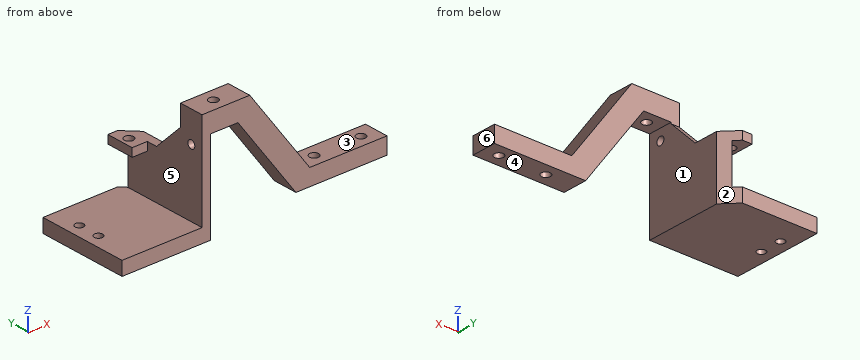
```python
from build123d import *

# Parameters (mm, degrees)
SZKIC1_W                    = 28
SZKIC1_H                    = 9
SZKIC1_R                    = 1.65
DODANIE_WYCI_GNI_CIE1_DEPTH = 6
DODANIE_WYCI_GNI_CIE2_DEPTH = 9
SZKIC3_W                    = 3
SZKIC3_H                    = 40.009031977
DODANIE_WYCI_GNI_CIE3_DEPTH = 9
SZKIC10_R                   = 1.65
WYTNIJ_WYCI_GNI_CIE4_DEPTH  = 7
SZKIC11_W                   = 32
SZKIC11_H                   = 33
SZKIC11_R                   = 1.5
DODANIE_WYCI_GNI_CIE4_DEPTH = 5
SZKIC12_W                   = 3
SZKIC12_H                   = 17.504515989
DODANIE_WYCI_GNI_CIE5_DEPTH = 24
SZKIC13_W                   = 10
SZKIC13_H                   = 3
DODANIE_WYCI_GNI_CIE6_DEPTH = 33
SZKIC14_R                   = 1.65
WYTNIJ_WYCI_GNI_CIE5_DEPTH  = 3
SZKIC15_W                   = 7
SZKIC15_H                   = 22.85
WYTNIJ_WYCI_GNI_CIE6_DEPTH  = 3
SFAZOWANIE1_SIZE            = 10
SZKIC16_R                   = 1.5
WYTNIJ_WYCI_GNI_CIE7_DEPTH  = 5
SZKIC17_R                   = 1.46285789
WYTNIJ_WYCI_GNI_CIE8_DEPTH  = 3
SZKIC18_W                   = 3
SZKIC18_H                   = 10.15
WYTNIJ_WYCI_GNI_CIE9_DEPTH  = 1.5
WYTNIJ_WYCI_GNI_CIE10_REACH = 87.52


with BuildPart() as part:
    # Szkic1 → Dodanie-wyciągnięcie1 (new body)
    with BuildSketch(Plane.XY):
        with Locations((14, 4.5)):
            Rectangle(SZKIC1_W, SZKIC1_H)
        with Locations((5.5, 4.5)):
            Circle(SZKIC1_R, mode=Mode.SUBTRACT)
        with Locations((22.5, 4.5)):
            Circle(SZKIC1_R, mode=Mode.SUBTRACT)
    extrude(amount=DODANIE_WYCI_GNI_CIE1_DEPTH)

    # Szkic2 → Dodanie-wyciągnięcie2 (add)
    with BuildSketch(Plane.XZ):
        Polygon((0, 0), (-5, 0), (-26, 29.009031977), (-36, 29.009031977), (-36, 36.009031977), (-21.72391247, 36.009031977), (0, 6), align=None)
    extrude(amount=-DODANIE_WYCI_GNI_CIE2_DEPTH)

    # Szkic3 → Dodanie-wyciągnięcie3 (add)
    with BuildSketch(Plane.XZ):
        with Locations((-37.5, 16.004515988)):
            Rectangle(SZKIC3_W, SZKIC3_H)
    extrude(amount=-DODANIE_WYCI_GNI_CIE3_DEPTH)

    # Szkic10 → Wytnij-wyciągnięcie4 (cut)
    with BuildSketch(Plane.XY.offset(36.009031977)):
        with Locations((-31, 4.5)):
            Circle(SZKIC10_R)
    extrude(amount=-WYTNIJ_WYCI_GNI_CIE4_DEPTH, mode=Mode.SUBTRACT)

    # Szkic11 → Dodanie-wyciągnięcie4 (add)
    with BuildSketch(Plane(origin=(0, 0, -4), x_dir=(-1, 0, 0), z_dir=(0, 0, -1))):
        with Locations((52, 16.5)):
            Rectangle(SZKIC11_W, SZKIC11_H)
        with Locations((63.5, 15)):
            Circle(SZKIC11_R, mode=Mode.SUBTRACT)
    extrude(amount=-DODANIE_WYCI_GNI_CIE4_DEPTH)

    # Szkic12 → Dodanie-wyciągnięcie5 (add)
    with BuildSketch(Plane(origin=(0, 9, 0), x_dir=(1, 0, 0), z_dir=(0, 1, 0))):
        with Locations((-37.5, -9.752257995)):
            Rectangle(SZKIC12_W, SZKIC12_H)
    extrude(amount=DODANIE_WYCI_GNI_CIE5_DEPTH)

    # Szkic13 → Dodanie-wyciągnięcie6 (add)
    with BuildSketch(Plane(origin=(0, 33, 0), x_dir=(1, 0, 0), z_dir=(0, 1, 0))):
        with Locations((-41, -17.004515989)):
            Rectangle(SZKIC13_W, SZKIC13_H)
    extrude(amount=-DODANIE_WYCI_GNI_CIE6_DEPTH)

    # Szkic14 → Wytnij-wyciągnięcie5 (cut)
    with BuildSketch(Plane.XY.offset(18.504515989)):
        with Locations((-41.65, 27.5)):
            Circle(SZKIC14_R)
    extrude(amount=-WYTNIJ_WYCI_GNI_CIE5_DEPTH, mode=Mode.SUBTRACT)

    # Szkic15 → Wytnij-wyciągnięcie6 (cut)
    with BuildSketch(Plane.XY.offset(18.504515989)):
        with Locations((-42.5, 11.425)):
            Rectangle(SZKIC15_W, SZKIC15_H)
    extrude(amount=-WYTNIJ_WYCI_GNI_CIE6_DEPTH, mode=Mode.SUBTRACT)

    # Sfazowanie1
    sfazowanie1_edges = [part.edges().sort_by_distance(p)[0] for p in [
        (-37.5, 9, 18.504515989),
    ]]
    chamfer(sfazowanie1_edges, length=SFAZOWANIE1_SIZE)

    # Szkic16 → Wytnij-wyciągnięcie7 (cut)
    with BuildSketch(Plane.XY.offset(1)):
        with Locations((-63.5, 23)):
            Circle(SZKIC16_R)
    extrude(amount=-WYTNIJ_WYCI_GNI_CIE7_DEPTH, mode=Mode.SUBTRACT)

    # Szkic17 → Wytnij-wyciągnięcie8 (cut)
    with BuildSketch(Plane.ZY.offset(39)):
        with Locations((25.009031977, 4.5)):
            Circle(SZKIC17_R)
    extrude(amount=-WYTNIJ_WYCI_GNI_CIE8_DEPTH, mode=Mode.SUBTRACT)

    # Szkic18 → Wytnij-wyciągnięcie9 (cut)
    with BuildSketch(Plane.ZY.offset(46)):
        with Locations((17.004515989, 27.925)):
            Rectangle(SZKIC18_W, SZKIC18_H)
    extrude(amount=-WYTNIJ_WYCI_GNI_CIE9_DEPTH, mode=Mode.SUBTRACT)

    # Wytnij-wyciągnięcie10: up to this face of the body (flat: up to its plane)
    wytnij_wyci_gni_cie10_end = Plane(part.part.faces().sort_by_distance((-39.760074004, 27.060059494, 18.504515989))[0])
    # Szkic19 → Wytnij-wyciągnięcie10 (cut, up to the picked face)
    with BuildSketch(Plane(origin=(0, 0, -4), x_dir=(-1, 0, 0), z_dir=(0, 0, -1)), mode=Mode.PRIVATE) as wytnij_wyci_gni_cie10_sk1:
        Polygon((36, 28), (41, 33), (36, 33), align=None)
    wytnij_wyci_gni_cie10_tool1 = split(extrude(wytnij_wyci_gni_cie10_sk1.sketch, amount=-WYTNIJ_WYCI_GNI_CIE10_REACH, mode=Mode.PRIVATE), bisect_by=wytnij_wyci_gni_cie10_end, keep=Keep.BOTH, mode=Mode.PRIVATE)
    add(wytnij_wyci_gni_cie10_tool1.solids().sort_by(Axis((-37.666667, 31.333333, -4), (0, 0, 1)))[0], mode=Mode.SUBTRACT)


solid = part.part
```
Input: part model. Units: mm. Frame: model coordinates. Face numbers are marked on the shaded views. A direction names the side the tool comes from. Coordinates: 2 decimals unless noted, no trailing zeros. Write each loop counter-clockwise with the first axis right and the second up, starting at its lowest first coordinate (ties: lowest second). Pieces come first, ordered by that corner, then holes.
1) Section D-D on x = 5.5. Output: boundary loops of the cut face in (y, z).
2) Set-up query: the marked faces 1 and 2. Return all of +Z, -Z, +X, -X, +Y, -Y with unobstructed straight access to the full face (end or side cutting, diameter ignored); none if empty.
3) Material intervals for line 1 along Y through (x, z) = (-31, 33.5); line 2 along X through (y, z) = (4, 3); line 3 along Z through (x, y) = (-59, 6.5), sorted ascending.
4) Pin query (flat end, axial travel): pin 1 Ø3 at (x, z) = (-16, 22) entering from -Y; pin 2 Ø4 at (x, y) = (22.5, 4.5) entering from -Z; pin 3 Ø2.5 at (y, z) = (4.5, 25.01) entering from -X; pin 4 Ø2.5 at (x, y) = (-39, 28) entering from +Z. Return the tip coordinate at first contact, or that it passes through.
5) Section A-A on x = -63.5. Output: boundary loops of the cut face in (y, z), and give its area (3 significant figures).
6) Section B-B on z = 14.5. Output: boundary loops of the cut face in (x, y).
7) Mould query, pull axis Z, two halves, no side actions, for the marked faces 3, 4, 5 and 6. Classes: pulls with the +Z half, pulls with the -Z half, needs draft (parallel to the pull), parting line crosses it, or undercut.
8) Section C-C on y = 4.5. Output: boundary loops of the cut face in (x, z), and give its area (3 significant figures).
Check result:
1. outline: (0, 0) - (2.85, 0) - (2.85, 6) - (0, 6) - close; (6.15, 0) - (9, 0) - (9, 6) - (6.15, 6) - close
2. face 1: -Z, +Y, -Y
2. face 2: +Z, -Z, +X, +Y
3. line 1: y = 0 to 2.85, 6.15 to 9
3. line 2: x = -39 to -36, -7.17 to 3.93, 7.07 to 20.93, 24.07 to 28
3. line 3: z = -4 to 1
4. pin 1: stops at y = 0
4. pin 2: stops at z = 0
4. pin 3: stops at x = -24.01
4. pin 4: stops at z = 18.5
5. outline: (0, -4) - (13.5, -4) - (13.5, 1) - (0, 1) - close; (16.5, -4) - (21.5, -4) - (21.5, 1) - (16.5, 1) - close; (24.5, -4) - (33, -4) - (33, 1) - (24.5, 1) - close
5. area: 135 mm2
6. outline: (-39, 0) - (-36, 0) - (-36, 28) - (-39, 31) - close; (-15.5, 0) - (-6.15, 0) - (-6.15, 9) - (-15.5, 9) - close
7. face 3: pulls with the +Z half
7. face 4: pulls with the -Z half
7. face 5: undercut
7. face 6: needs draft
8. outline: (-68, -4) - (-36, -4) - (-36, 23.55) - (-39, 23.55) - (-39, 1) - (-68, 1) - close; (-39, 26.47) - (-36, 26.47) - (-36, 29.01) - (-32.65, 29.01) - (-32.65, 36.01) - (-39, 36.01) - close; (-29.35, 29.01) - (-26, 29.01) - (-5, 0) - (3.85, 0) - (3.85, 6) - (0, 6) - (-21.72, 36.01) - (-29.35, 36.01) - close; (7.15, 0) - (20.85, 0) - (20.85, 6) - (7.15, 6) - close; (24.15, 0) - (28, 0) - (28, 6) - (24.15, 6) - close
8. area: 737 mm2
